from build123d import *

# Parameters (mm, degrees)
F1_DEPTH = 381


with BuildPart() as f1:
    # F0 (on Right) → F1 (new body)
    with BuildSketch(Plane.YZ):
        with BuildLine():
            Line((4.474148, 167.432852), (-59.025852, 167.432852))
            Line((-59.025852, 167.432852), (-59.025852, 0))
            Line((-59.025852, 0), (-59.025852, -84.542013))
            Line((-59.025852, -84.542013), (1007.774148, -84.542013))
            Line((1007.774148, -84.542013), (1007.774148, 0))
            Line((1007.774148, 0), (1007.774148, 69.85))
            ThreePointArc((1007.774148, 69.85), (846.327713, 17.653603), (677.574148, 0))
            ThreePointArc((677.574148, 0), (330.768233, 42.486428), (4.474148, 167.432852))
        make_face()
    extrude(amount=F1_DEPTH)


solid = f1.part
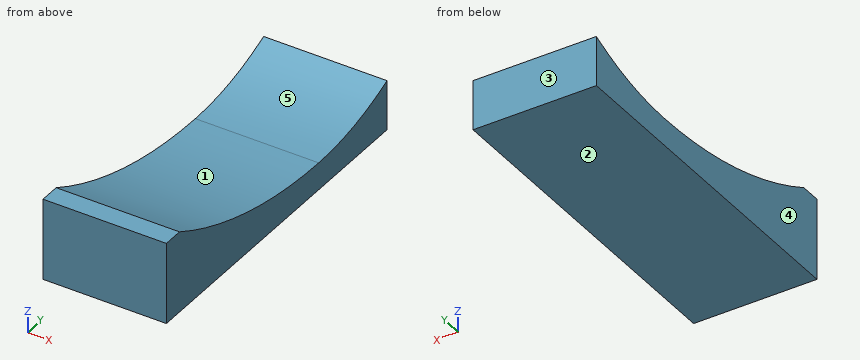
Build history of the part. All positions in model axes, mm. Face numbers are marked on the shaded views. A direction names the side the tool comes from. Give positions to 0.01 mm unless a question says otherwise; leave off trailing zeros. Loops run counter-clockwise (first coordinate to the right, second up) from the corner with the lowest first, then second, coordinate; pieces in that order, holes last. Notation, with made-up numbers: (-16, -36) - (3, -36) arc R19 ccw to (3, -11) - close; hole circle Ø9 at (18.5, 46.5). An arc over 180 degrees is marked (long way). Write item = value, one per line. Start each with the question number.
1) Band-saw the part on C-C on y = 367.5. Give the cut face in (x, z), plus the area to 3 significant figures.
2) Band-saw the part on D-D on z = 131. Give the cut face in (x, y), plus the area to 3 significant figures.
3) Pull direction Y, two halves, no side cores. Call the marked faces 1, 2 and 3: +Y half, -Y half, draft (parallel to the pull), parting line (faces both ways), or undercut.
4) Band-saw the part on A-A on z = 15. Give the cut face in (x, y), plus the area to 3 significant figures.
5) Tool access for the marked faces 4 and 5: list every direction of +Z, -Z, +X, -X, +Y, -Y with a clear straight run to the whole face (end or side of a thin tool).
6) Drop flat-ended pins along their axis: pin 1 Ø5 at (x, y) = (316, 248.5) entering from +Z; pin 2 Ø10 at (x, y) = (288, 887) entering from +Z. Give the stop position or say it passes through.
7) Probe probe 1 along Z at (x, y) = (139.5, 824.5); probe 2 along Z at (x, y) = (35.5, 495.5); probe 3 along Y at (x, z) = (365.5, 112.5). List the from-to ranges inside material, lowest first. Write a range as from..to.
Final values:
q1.outline = (0, -84.54) - (381, -84.54) - (381, 33.86) - (0, 33.86) - close
q1.area = 45,100 mm²
q2.outline = (0, -59.03) - (381, -59.03) - (381, 78.2) - (0, 78.2) - close
q2.area = 52,300 mm²
q3.face_1 = undercut
q3.face_2 = draft
q3.face_3 = +Y half
q4.outline = (0, -59.03) - (381, -59.03) - (381, 470.51) - (0, 470.51) - close; (0, 833.26) - (381, 833.26) - (381, 1007.77) - (0, 1007.77) - close
q4.area = 268,000 mm²
q5.face_4 = +Z, -Z, -X, +Y, -Y
q5.face_5 = +Z, +X, -X
q6.pin_1 = 66.35
q6.pin_2 = 28.7
q7.probe_1 = -84.54..13.35
q7.probe_2 = -84.54..11.58
q7.probe_3 = -59.03..120.26
